Part model, mm, in its own coordinate system. A direction names the side the tool comes from. Round coordinates to 2 decimals unless told otherwise and drop trailing zeros. Write each loop counter-clockwise with the first axis right and the second up, starting at its lowest first coordinate (ties: lowest second). Pieces come first, ordered by that corner, then holes.
```python
from build123d import *

# Parameters (mm, degrees)
SKETCH1_W            = 45
SKETCH1_H            = 25.5
SKETCH1_W_2          = 41
SKETCH1_H_2          = 21.5
BOSS_EXTRUDE1_DEPTH  = 15
SKETCH2_W            = 48
SKETCH2_H            = 28.5
SKETCH2_W_2          = 37
SKETCH2_H_2          = 17.5
BOSS_EXTRUDE2_DEPTH  = 3
FILLET1_R            = 0.5
FILLET2_R            = 0.5
CHAMFER1_SIZE        = 2
FILLET3_R            = 0.5
SKETCH3_W            = 39
SKETCH3_H            = 19.5
BOSS_EXTRUDE3_DEPTH  = 0.1
SKETCH4_W            = 2
SKETCH4_H            = 5.5
CUT_EXTRUDE1_DEPTH   = 7
BOSS_EXTRUDE4_DEPTH  = 2
SKETCH6_W            = 25
SKETCH6_H            = 8
CUT_EXTRUDE4_DEPTH   = 2
BOSS_EXTRUDE5_DEPTH  = 9
MIRROR5_COPY_1_DEPTH = 9


with BuildPart() as part:
    # Sketch1 → Boss-Extrude1 (new body)
    with BuildSketch(Plane.XY):
        with Locations((22.5, 12.75)):
            Rectangle(SKETCH1_W, SKETCH1_H)
        with Locations((22.5, 12.75)):
            Rectangle(SKETCH1_W_2, SKETCH1_H_2, mode=Mode.SUBTRACT)
    extrude(amount=BOSS_EXTRUDE1_DEPTH)

    # Sketch2 → Boss-Extrude2 (add)
    with BuildSketch(Plane.XY.offset(15)):
        with Locations((22.5, 12.75)):
            Rectangle(SKETCH2_W, SKETCH2_H)
        with Locations((22.5, 12.75)):
            Rectangle(SKETCH2_W_2, SKETCH2_H_2, mode=Mode.SUBTRACT)
    extrude(amount=BOSS_EXTRUDE2_DEPTH)

    # Fillet1
    fillet1_edges = [part.edges().sort_by_distance(p)[0] for p in [
        (46.5, -1.5, 16.5),
        (46.5, 27, 16.5),
        (-1.5, 27, 16.5),
        (-1.5, -1.5, 16.5),
    ]]
    fillet(fillet1_edges, radius=FILLET1_R)

    # Fillet2
    fillet2_edges = [part.edges().sort_by_distance(p)[0] for p in [
        (22.5, 27, 18),
        (46.5, 12.75, 18),
        (-1.5, 12.75, 18),
        (22.5, -1.5, 18),
        (-1.353553391, 26.853553391, 18),
        (-1.353553391, -1.353553391, 18),
        (46.353553391, -1.353553391, 18),
        (46.353553391, 26.853553391, 18),
    ]]
    fillet(fillet2_edges, radius=FILLET2_R)

    # Chamfer1
    chamfer1_edges = [part.edges().sort_by_distance(p)[0] for p in [
        (41, 12.75, 18),
        (22.5, 21.5, 18),
        (4, 12.75, 18),
        (22.5, 4, 18),
    ]]
    chamfer(chamfer1_edges, length=CHAMFER1_SIZE)

    # Fillet3
    fillet3_edges = [part.edges().sort_by_distance(p)[0] for p in [
        (22.5, 2, 18),
        (2, 12.75, 18),
        (22.5, 23.5, 18),
        (43, 12.75, 18),
    ]]
    fillet(fillet3_edges, radius=FILLET3_R)

    # Sketch3 → Boss-Extrude3 (add)
    with BuildSketch(Plane(origin=(0, 0, 15), x_dir=(-1, 0, 0), z_dir=(0, 0, -1))):
        with Locations((-22.5, 12.75)):
            Rectangle(SKETCH3_W, SKETCH3_H)
    extrude(amount=BOSS_EXTRUDE3_DEPTH)

    # Sketch4 → Cut-Extrude1 (cut)
    with BuildSketch(Plane.ZY):
        Polygon((0, 25.5), (0, 23.5), (11.354344123, 23.5), (11.354344123, 22.2), (3.354344123, 22.2), (3.354344123, 21.5), (-1.052747885, 21.5), (-1.052747885, 19.2), (11.35, 19.2), (11.35, 16.2), (-2.740421073, 16.2), (-2.133707004, 24.508604023), align=None)
        Polygon((-2.133707004, 0.991395977), (0, 0), (0, 2), (11.354344123, 2), (11.354344123, 3.3), (3.354344123, 3.3), (3.354344123, 4), (-1.052747885, 4), (-1.052747885, 6.3), (11.35, 6.3), (11.35, 9.3), (-2.740421073, 9.3), align=None)
        with Locations((6, 12.75)):
            Rectangle(SKETCH4_W, SKETCH4_H)
    cut_extrude1 = extrude(amount=-CUT_EXTRUDE1_DEPTH, mode=Mode.SUBTRACT)

    # Mirror1: Cut-Extrude1 across plane
    add(cut_extrude1.mirror(Plane(origin=(22.5, 0, 0), x_dir=(0, 0, 1), z_dir=(1, 0, 0))), mode=Mode.SUBTRACT)

    # Sketch5 → Boss-Extrude4 (add)
    with BuildSketch(Plane.ZY):
        with BuildLine():
            Line((0, 21.5), (-2.205642109, 23.044407231))
            ThreePointArc((-2.205642109, 23.044407231), (-2.462636709, 23.13394276), (-2.728457708, 23.075615822))
            Line((-2.728457708, 23.075615822), (-3.522154827, 22.650614026))
            ThreePointArc((-3.522154827, 22.650614026), (-3.745020462, 22.408367067), (-3.768996943, 22.08007176))
            Line((-3.768996943, 22.08007176), (-3.504631096, 21.096282354))
            ThreePointArc((-3.504631096, 21.096282354), (-3.431234223, 20.939104177), (-3.308549817, 20.816463984))
            Line((-3.308549817, 20.816463984), (-1.129138824, 19.290423978))
            ThreePointArc((-1.129138824, 19.290423978), (-0.992703505, 19.223141525), (-0.842350606, 19.2))
            Line((-0.842350606, 19.2), (0, 19.2))
            Line((0, 19.2), (0, 21.5))
        make_face()
        with BuildLine():
            Line((-3.522154827, 2.849385974), (-2.728457708, 2.424384178))
            ThreePointArc((-2.728457708, 2.424384178), (-2.462636709, 2.36605724), (-2.205642109, 2.455592769))
            Line((-2.205642109, 2.455592769), (0, 4))
            Line((0, 4), (0, 6.3))
            Line((0, 6.3), (-0.842350606, 6.3))
            ThreePointArc((-0.842350606, 6.3), (-0.992703505, 6.276858475), (-1.129138824, 6.209576022))
            Line((-1.129138824, 6.209576022), (-3.308549817, 4.683536016))
            ThreePointArc((-3.308549817, 4.683536016), (-3.431234223, 4.560895823), (-3.504631096, 4.403717646))
            Line((-3.504631096, 4.403717646), (-3.768996943, 3.41992824))
            ThreePointArc((-3.768996943, 3.41992824), (-3.745020462, 3.091632933), (-3.522154827, 2.849385974))
        make_face()
    boss_extrude4 = extrude(amount=-BOSS_EXTRUDE4_DEPTH)

    # Mirror3: Boss-Extrude4 across plane
    add(boss_extrude4.mirror(Plane(origin=(22.5, 0, 0), x_dir=(0, 0, 1), z_dir=(1, 0, 0))))

    # Sketch6 → Cut-Extrude4 (cut)
    with BuildSketch(Plane(origin=(0, 25.5, 0), x_dir=(1, 0, 0), z_dir=(0, 1, 0))):
        with Locations((22.5, -11)):
            Rectangle(SKETCH6_W, SKETCH6_H)
    cut_extrude4 = extrude(amount=-CUT_EXTRUDE4_DEPTH, mode=Mode.SUBTRACT)

    # Sketch7 → Boss-Extrude5 (add)
    with BuildSketch(Plane(origin=(11, 0, 0), x_dir=(0, 0, -1), z_dir=(1, 0, 0))):
        with BuildLine():
            Line((-7, 23.5), (-13.5, 23.5))
            Line((-13.5, 23.5), (-13.5, 25.5))
            Line((-13.5, 25.5), (-12.50438631, 25.92802582))
            ThreePointArc((-12.50438631, 25.92802582), (-12.308138031, 25.84987504), (-12.229830148, 26.046060684))
            Line((-12.229830148, 26.046060684), (-11.58568767, 26.322984972))
            ThreePointArc((-11.58568767, 26.322984972), (-11.389415731, 26.244779249), (-11.311131441, 26.441019864))
            Line((-11.311131441, 26.441019864), (-10.666989007, 26.717944134))
            ThreePointArc((-10.666989007, 26.717944134), (-10.47069343, 26.639683459), (-10.392432756, 26.835979036))
            Line((-10.392432756, 26.835979036), (-9.545698193, 27.2))
            Line((-9.545698193, 27.2), (-8.3, 25.5))
            Line((-8.3, 25.5), (-7, 25.5))
            Line((-7, 25.5), (-7, 23.5))
        make_face()
    boss_extrude5 = extrude(amount=BOSS_EXTRUDE5_DEPTH)

    # Mirror4: Boss-Extrude5 across plane
    add(boss_extrude5.mirror(Plane(origin=(22.5, 0, 0), x_dir=(0, 0, 1), z_dir=(1, 0, 0))))

    # Mirror5: Cut-Extrude4, Boss-Extrude5 across plane
    add(cut_extrude4.mirror(Plane.ZX.offset(12.75)), mode=Mode.SUBTRACT)
    add(boss_extrude5.mirror(Plane.ZX.offset(12.75)))

    # Mirror5 copy 1 sketch → Mirror5 copy 1 (add)
    with BuildSketch(Plane(origin=(34, 25.5, 0), x_dir=(0, 0, -1), z_dir=(-1, 0, 0))):
        with BuildLine():
            Line((-7, 23.5), (-13.5, 23.5))
            Line((-13.5, 23.5), (-13.5, 25.5))
            Line((-13.5, 25.5), (-12.50438631, 25.92802582))
            ThreePointArc((-12.50438631, 25.92802582), (-12.308138031, 25.84987504), (-12.229830148, 26.046060684))
            Line((-12.229830148, 26.046060684), (-11.58568767, 26.322984972))
            ThreePointArc((-11.58568767, 26.322984972), (-11.389415731, 26.244779249), (-11.311131441, 26.441019864))
            Line((-11.311131441, 26.441019864), (-10.666989007, 26.717944134))
            ThreePointArc((-10.666989007, 26.717944134), (-10.47069343, 26.639683459), (-10.392432756, 26.835979036))
            Line((-10.392432756, 26.835979036), (-9.545698193, 27.2))
            Line((-9.545698193, 27.2), (-8.3, 25.5))
            Line((-8.3, 25.5), (-7, 25.5))
            Line((-7, 25.5), (-7, 23.5))
        make_face()
    extrude(amount=MIRROR5_COPY_1_DEPTH)


solid = part.part
```
Q1. Cut at D-D on x = 5. Write the cut outline in (y, z), plus the area to 3 significant figures.
Values follow:
outline: (-1.5, 15) - (0, 15) - (0, 0) - (2, 0) - (2, 15) - (3, 15) - (3, 14.9) - (22.5, 14.9) - (22.5, 15) - (23.5, 15) - (23.5, 0) - (25.5, 0) - (25.5, 15) - (27, 15) - (27, 17.5) arc R0.5 ccw to (26.5, 18) - (23.71, 18) arc R0.5 ccw to (23.35, 17.85) - (21.5, 16) - (21.5, 15) - (4, 15) - (4, 16) - (2.15, 17.85) arc R0.5 ccw to (1.79, 18) - (-1, 18) arc R0.5 ccw to (-1.5, 17.5) - close
area: 90.8 mm2
Q2. Cut at B-B on y = 8. Write the cut outline in (x, z).
Values follow:
outline: (-1.5, 15) - (0, 15) - (0, 11.35) - (2, 11.35) - (2, 15) - (3, 15) - (3, 14.9) - (42, 14.9) - (42, 15) - (43, 15) - (43, 11.35) - (45, 11.35) - (45, 15) - (46.5, 15) - (46.5, 17.5) arc R0.5 ccw to (46, 18) - (43.21, 18) arc R0.5 ccw to (42.85, 17.85) - (41, 16) - (41, 15) - (4, 15) - (4, 16) - (2.15, 17.85) arc R0.5 ccw to (1.79, 18) - (-1, 18) arc R0.5 ccw to (-1.5, 17.5) - close
Q3. Mould opens along Y. For faces 5 (the flat face through (1, 16.2, 6)), 6 (the flat face through (1, 9.3, 6)), 7 (the flat face through (29.56, -0.21, 13.01)), 8 (the flat face through (10, 25, 11)) say: +Y half, -Y half, draft (parallel to the pull), parting line (faces both ways), or undercut.
Values follow:
face 5: undercut
face 6: undercut
face 7: -Y half
face 8: draft
Q4. Drop flat-ended pins along their axis: pin 1 (1.5 mm diameter, centred on y = 8, z = 5, fed in from +X); pin 2 (0.6 mm diameter, centred on x = 0.5, z = 7, fed in from -Y); pin 3 (0.6 mm diameter, centred on x = 43.5, z = 3, fed in from +Y); pin 4 (1.6 mm diameter, centred on y = 1, z = 10.5, fed in from +X). Give the stop position or say it passes through.
Values follow:
pin 1: passes through
pin 2: stops at y = 0
pin 3: stops at y = 25.5
pin 4: stops at x = 45
Q5. Cut at A-A on z = 4.25. State how many separate pieces and enclosed holes the cut face has, plus the area to 3 significant figures.
Values follow:
separate pieces: 8
enclosed holes: 0
area: 232 mm2
Q6. Wall check: L1, parallel to X at y = 25, z = 12.25; L2, parallel to Y at x = 4.5, z = 4.25; L3, parallel to X at y = 13.5, z = 9.5. Give the ranges that are in metal, low to high.
Values follow:
L1: x = 0 to 10, 11 to 20, 25 to 34, 35 to 45
L2: y = 0 to 2, 23.5 to 25.5
L3: x = 0 to 2, 43 to 45
Q7. Which spindle directions (+Z, -Z, +X, -X, +Y, -Y) get a long thin tool onto all of the face, cutting with end or side? Do faces 1 (the flat face through (44.01, 5.46, -2.2)), 2 (the flat face through (34, 25, 10)), 3 (the flat face through (0.986, 22.261, -1.087)), 4 (the flat face through (1, 21.5, 2)). Say none if no direction does.
Values follow:
face 1: -Z, +X, -X
face 2: +Y, -Y
face 3: +X, -X, +Y
face 4: +X, -X
